```python
from build123d import *

# Parameters (mm, degrees)
SKETCH2_W           = 14.605
SKETCH2_H           = 7.62
BOSS_EXTRUDE1_DEPTH = 1.5875
SKETCH3_R           = 1.524
CUT_EXTRUDE1_DEPTH  = 68.907542479
FILLET1_R           = 0.508
FILLET2_R           = 6.604


with BuildPart() as part:
    # Sketch2 → Boss-Extrude1 (new body)
    with BuildSketch(Plane.XY):
        with BuildLine():
            Line((-2.286, 26.7335), (-2.286, 23.0505))
            Line((-2.286, 23.0505), (18.796, 23.0505))
            Line((18.796, 23.0505), (20.066, 23.0505))
            Line((20.066, 23.0505), (20.066, 32.5755))
            Line((20.066, 32.5755), (59.563, 32.5755))
            Line((59.563, 32.5755), (59.563, 13.462))
            Line((59.563, 13.462), (59.563, -13.462))
            Line((59.563, -13.462), (59.563, -32.5755))
            Line((59.563, -32.5755), (20.066, -32.5755))
            Line((20.066, -32.5755), (20.066, -23.0505))
            Line((20.066, -23.0505), (18.796, -23.0505))
            Line((18.796, -23.0505), (-2.286, -23.0505))
            Line((-2.286, -23.0505), (-2.286, -26.7335))
            ThreePointArc((-2.286, -26.7335), (-3.997082184, -30.864417816), (-8.128, -32.5755))
            Line((-8.128, -32.5755), (-12.7, -32.5755))
            ThreePointArc((-12.7, -32.5755), (-16.830917816, -30.864417816), (-18.542, -26.7335))
            Line((-18.542, -26.7335), (-18.542, 26.7335))
            ThreePointArc((-18.542, 26.7335), (-16.830917816, 30.864417816), (-12.7, 32.5755))
            Line((-12.7, 32.5755), (-8.128, 32.5755))
            ThreePointArc((-8.128, 32.5755), (-3.997082184, 30.864417816), (-2.286, 26.7335))
        make_face()
        with Locations((39.8145, -9.652)):
            Rectangle(SKETCH2_W, SKETCH2_H, mode=Mode.SUBTRACT)
        with Locations((39.8145, 9.652)):
            Rectangle(SKETCH2_W, SKETCH2_H, mode=Mode.SUBTRACT)
    extrude(amount=BOSS_EXTRUDE1_DEPTH)

    # Sketch3 → Cut-Extrude1 (cut, through all)
    with BuildSketch(Plane(origin=(0, 0, 0), x_dir=(-1, 0, 0), z_dir=(0, 0, -1))):
        with Locations((-53.34, 12.98575)):
            Circle(SKETCH3_R)
        with Locations(Location((-53.34, -12.98575, 0), (0, 0, 180))):
            Circle(SKETCH3_R)
        with Locations((-2.54, 20.6375)):
            Circle(SKETCH3_R)
        with Locations(Location((-2.54, -20.6375, 0), (0, 0, 180))):
            Circle(SKETCH3_R)
    extrude(amount=-CUT_EXTRUDE1_DEPTH, mode=Mode.SUBTRACT)

    # Fillet1
    fillet1_edges = [part.edges().sort_by_distance(p)[0] for p in [
        (-2.286, -23.0505, 0.79375),
        (-2.286, 23.0505, 0.79375),
        (20.066, 23.0505, 0.79375),
        (20.066, -23.0505, 0.79375),
        (32.512, 13.462, 0.79375),
        (32.512, 5.842, 0.79375),
        (47.117, 5.842, 0.79375),
        (47.117, 13.462, 0.79375),
        (47.117, -5.842, 0.79375),
        (32.512, -5.842, 0.79375),
        (32.512, -13.462, 0.79375),
        (47.117, -13.462, 0.79375),
    ]]
    fillet(fillet1_edges, radius=FILLET1_R)

    # Fillet2
    fillet2_edges = [part.edges().sort_by_distance(p)[0] for p in [
        (20.066, 32.5755, 0.79375),
        (59.563, 32.5755, 0.79375),
        (59.563, -32.5755, 0.79375),
        (20.066, -32.5755, 0.79375),
    ]]
    fillet(fillet2_edges, radius=FILLET2_R)


solid = part.part
```
The listing builds one solid part. Answer for the finished solid, in the listing's coordinates (mm). A direction names the side the tool comes from. Round coordinates to 2 decimals unless told otherwise and drop trailing zeros. Order: outer loops, then holes, each group sorted by start corner. A loop starts at its lowest first (then second) coordinate and runs counter-clockwise, first axis right, second up. Notation, with made-up numbers: (65.5, 19.5) - (106.5, 19.5) arc R19 cw to (106.5, 36.5) - close; hole circle Ø8 at (29, 55.5). An arc over 180 degrees is marked (long way). Put each result on its own line as item: value. Start each with the question number.
(1) Find section C-C (y = 7.5). Give the vertices of the cut face in (x, z).
(2) Find section B-B (x = 2.54). Give the vertices of the cut face in (y, z), plus the area to 3 significant figures.
(3) For faces 4 (the cylindrical face through (-4.043, 30.91, 0.783)), 5 (the flat face through (20.066, -25, 1)), 6 (the flat face through (47.117, 10, 1)), determine the directions among +Z, -Z, +X, -X, +Y, -Y from which every point of the face is accessible in a straight line to the end or side of a thin tool.
(4) Find section A-A (y = 25). Give the vertices of the cut face in (x, z).
(5) Straight lines are drawn through the part: probe 1 along Y at (x, z) = (2.54, 0.7); probe 2 along Y at (x, z) = (53.34, 0.6); probe 3 along Y at (x, z) = (11.5, 1.25). For each, find the intervals that lie inside material, in ascending order. Write a range as from..to.
(6) Determine the mould class of faces 1 (the cylindrical face through (52.52, 14.27, 0.78)), 2 (the flat face through (40, -32.575, 1)), 3 (the flat face through (-10, 32.575, 1)) for opening direction Y: released by +Y, released by -Y, zero draft, split by the parting line, or undercut.
(7) Given P1, Ø3.5, axis at x = 2.54, y = -20.64, coming from the -Z side, flat-ended and moving along its own axis, determine where the tip first touches the part or whether it passes through.
(8) Find section D-D (z = 0.65). State how many separate pieces and enclosed holes the cut face has, plus the area to 3 significant figures.
Reply:
1. outline: (-18.54, 0) - (32.51, 0) - (32.51, 1.59) - (-18.54, 1.59) - close; (47.12, 0) - (59.56, 0) - (59.56, 1.59) - (47.12, 1.59) - close
2. outline: (-23.05, 0) - (-22.16, 0) - (-22.16, 1.59) - (-23.05, 1.59) - close; (-19.11, 0) - (19.11, 0) - (19.11, 1.59) - (-19.11, 1.59) - close; (22.16, 0) - (23.05, 0) - (23.05, 1.59) - (22.16, 1.59) - close
2. area: 63.5 mm^2
3. face 4: +Z, -Z, +Y
3. face 5: +Z, -Z, -Y
3. face 6: +Z, -Z
4. outline: (-18.54, 0) - (-2.29, 0) - (-2.29, 1.59) - (-18.54, 1.59) - close; (20.07, 0) - (59.56, 0) - (59.56, 1.59) - (20.07, 1.59) - close
5. probe 1: -23.05..-22.16, -19.11..19.11, 22.16..23.05
5. probe 2: -32.56..-14.51, -11.46..11.46, 14.51..32.56
5. probe 3: -23.05..23.05
6. face 1: undercut
6. face 2: released by -Y
6. face 3: released by +Y
7. P1: z = 0
8. separate pieces: 1
8. enclosed holes: 6
8. area: 4,340 mm^2
